Input: part model. Units: mm. Frame: model coordinates. A direction names the side the tool comes from. Round coordinates to 2 decimals unless told otherwise and drop trailing zeros. Write each loop counter-clockwise with the first axis right and the second up, starting at its lowest first coordinate (ties: lowest second). Pieces come first, ordered by that corner, then holes. Notation, with made-up numbers: (82, 24) -> (86, 24) arc R23 ccw to (86, 49) -> close; hole circle Ø2 at (15.25, 23). An arc over 180 degrees is marked (long way). Write item = value, one per line. Start each with the question number.
```python
from build123d import *

# Parameters (mm, degrees)
SKETCH1_R                = 6.35
BOSS_EXTRUDE1_DEPTH      = 12.7
BOSS_EXTRUDE2_DEPTH      = 19.05
BOSS_EXTRUDE2_DEPTH_BACK = 31.75
SKETCH2_R                = 3.175
CUT_EXTRUDE1_START       = -2.54
SKETCH3_OUTSIDE_W        = 247.57
SKETCH3_OUTSIDE_H        = 76.12
SKETCH3_OUTSIDE_R        = 2.54
CUT_EXTRUDE1_DEPTH       = 16.51
CUT_EXTRUDE2_START       = -2.54
SKETCH4_OUTSIDE_W        = 247.57
SKETCH4_OUTSIDE_H        = 76.12
SKETCH4_OUTSIDE_R        = 2.54
CUT_EXTRUDE2_DEPTH       = 16.51
REVOLVE1_ANGLE           = 180
SKETCH9_W                = 4.061831886
SKETCH9_H                = 0.660529679
BOSS_EXTRUDE4_DEPTH      = 10.16


with BuildPart() as part:
    # Sketch1 → Boss-Extrude1 (new body)
    with BuildSketch(Plane.XY):
        with BuildLine():
            Line((16.512967167, -9.984929936), (16.512967167, -41.734929936))
            Line((16.512967167, -41.734929936), (-170.812032833, -41.734929936))
            ThreePointArc((-170.812032833, -41.734929936), (-186.687032833, -25.859929936), (-170.812032833, -9.984929936))
            Line((-170.812032833, -9.984929936), (16.512967167, -9.984929936))
        make_face()
        with Locations((-116.837032833, -25.859929936)):
            Circle(SKETCH1_R, mode=Mode.SUBTRACT)
    extrude(amount=BOSS_EXTRUDE1_DEPTH)

    # Sketch2 → Boss-Extrude2 (add, two sides: drawn at the far end of the back side and taken through both)
    with BuildSketch(Plane.XY.offset(12.7).offset(-BOSS_EXTRUDE2_DEPTH_BACK)):
        with Locations((-167.637032833, -25.859929936)):
            Circle(SKETCH2_R)
    extrude(amount=BOSS_EXTRUDE2_DEPTH + BOSS_EXTRUDE2_DEPTH_BACK)

    # Sketch3 outside → Cut-Extrude1 (cut)
    with BuildSketch(Plane.XY.offset(31.75).offset(CUT_EXTRUDE1_START)):
        with Locations((-85.087, -25.86)):
            Rectangle(SKETCH3_OUTSIDE_W, SKETCH3_OUTSIDE_H)
        with Locations((-167.637032833, -25.859929936)):
            Circle(SKETCH3_OUTSIDE_R, mode=Mode.SUBTRACT)
    extrude(amount=-CUT_EXTRUDE1_DEPTH, mode=Mode.SUBTRACT)

    # Sketch4 outside → Cut-Extrude2 (cut)
    with BuildSketch(Plane(origin=(0, 0, -19.05), x_dir=(-1, 0, 0), z_dir=(0, 0, -1)).offset(CUT_EXTRUDE2_START)):
        with Locations((85.087, -25.86)):
            Rectangle(SKETCH4_OUTSIDE_W, SKETCH4_OUTSIDE_H)
        with Locations(Location((167.637032833, -25.859929936, 0), (0, 0, 180))):
            Circle(SKETCH4_OUTSIDE_R, mode=Mode.SUBTRACT)
    extrude(amount=-CUT_EXTRUDE2_DEPTH, mode=Mode.SUBTRACT)

    # Sketch6 → Revolve1 (revolve)
    with BuildSketch(Plane(origin=(16.512967167, 0, 0), x_dir=(0, 0, -1), z_dir=(1, 0, 0))):
        with BuildLine():
            Line((-6.35, -9.984929936), (-6.35, -41.734929936))
            ThreePointArc((-6.35, -41.734929936), (-22.245527261, -25.859929936), (-6.35, -9.984929936))
        make_face()
    revolve(axis=Axis((16.512967167, -9.984929936, 6.35), (0, 1, 0)), revolution_arc=REVOLVE1_ANGLE)

    # Sketch9 → Boss-Extrude4 (add)
    with BuildSketch(Plane.XY.offset(12.7)):
        with Locations((-167.595763161, -28.664448748)):
            Rectangle(SKETCH9_W, SKETCH9_H)
    extrude(amount=BOSS_EXTRUDE4_DEPTH)


solid = part.part
```
1. Line query: line 1 along Z through (x, y) = (-52.5, -21); line 2 along Y through (x, z) = (-116, 0.5); line 3 along X through (y, z) = (-27, -4). Output: solid intervals per line, ascending.
2. Section B-B (x = -20.5). Output: boundary loops of the cut face in (y, z).
3. Section A-A (x = -116). Output: boundary loops of the cut face in (y, z).
4. Reachability of faces 1 (the flat face through (-168, -26, 31.75)), 2 (the cylindrical face through (-170.81, -25.72, -17.8)), 3 (the flat face through (16.513, -26, -4)), 4 (the cylindrical face through (-166.3, -23.7, 21.1)) from +Z, -Z, +X, -X, +Y, -Y: full face, straight path, thin tool, end or side. Return the list, or none.
5. Mould query, pull axis X, two halves, no side actions, for faces 5 (the flat face through (16.513, -26, 16)), 6 (the flat face through (-165, -27, -16.51)), 7 (the cylindrical face through (-170.81, -25.72, 30.46)). Classes: pulls with the +X half, pulls with the -X half, needs draft (parallel to the pull), parting line crosses it, or undercut.
6. Pin query (flat end, axial travel): P1, Ø8, axis at x = -95.5, y = -22, coming from the -Z side; P2, Ø7.5, axis at y = -32.5, z = 18.5, coming from the -X side; P3, Ø4, axis at y = -24.5, z = 19, coming from the -X side. Return the tip coordinate at first contact, or that it passes through.
Check sheet entries:
q1.line_1 = 0 to 12.7
q1.line_2 = -41.73 to -32.15, -19.57 to -9.98
q1.line_3 = -169.91 to -165.37, 16.51 to 28.52
q2.outline = (-41.73, 0) -> (-9.98, 0) -> (-9.98, 12.7) -> (-41.73, 12.7) -> close
q3.outline = (-41.73, 0) -> (-32.15, 0) -> (-32.15, 12.7) -> (-41.73, 12.7) -> close; (-19.57, 0) -> (-9.98, 0) -> (-9.98, 12.7) -> (-19.57, 12.7) -> close
q4.face_1 = +Z, +X, -X, +Y, -Y
q4.face_2 = -Z
q4.face_3 = -Z, +Y, -Y
q4.face_4 = none
q5.face_5 = undercut
q5.face_6 = needs draft
q5.face_7 = parting line crosses it
q6.P1 = 0
q6.P2 = -169.63
q6.P3 = -170.18
